Geometry: final body of the model. Coordinates: model frame, mm. Face numbers are marked on the shaded views. A direction names the side the tool comes from. Coordinates: 2 decimals unless noted, no trailing zeros. Order: outer loops, then holes, each group sorted by start corner. A loop starts at its lowest first (then second) coordinate and runs counter-clockwise, first axis right, second up. Notation, with made-up numbers: M 86.5,74 L 92.5,74 A20 ccw 92.5,98 Z; hole C 21,-1 d7. An arc over 180 degrees is marked long. Use CSV: the item, a comma, the result in double quotes. Start each with the question number.
1. First-contact query: P1, Ø17, axis at x = -33.5, y = 3, coming from the +Z side; P2, Ø6, axis at x = 8, z = 20, coming from the +Y side; P3, Ø1.5, axis at y = 3.5, z = 1.5, coming from the -X side; P4, Ø3, axis at x = 20, y = 3.05, coming from the +Z side. Flat tips, straight axial feed; report the tip coordinate or a pass-through.
2. Section query A-A on x = -20. Return the cut outline in (y, z).
3. Section query B-B on y = 7. Return the cut outline in (x, z).
4. Set-up query: the marked faces 1, 2 and 3. Return all of +Z, -Z, +X, -X, +Y, -Y with unobstructed straight access to the full face (end or side cutting, diameter ignored); none if empty.
5. Section query D-D on x = 31.5. Return the cut outline in (y, z).
6. Material intervals for line 1 (Y direction, x = 20, z = 3.5); line 2 (Y direction, x = -20, z = 3.8); line 3 (X direction, y = 20, z = 30), sorted ascending.
7. Section query C-C on z = 7.5. Return the cut outline in (x, y).
8. Pull-direction query (X, two-part tool) for the marked faces 4, 5 and 6; classes: pulls with the +X half, pulls with the -X half, needs draft (parallel to the pull), parting line crosses it, or undercut.
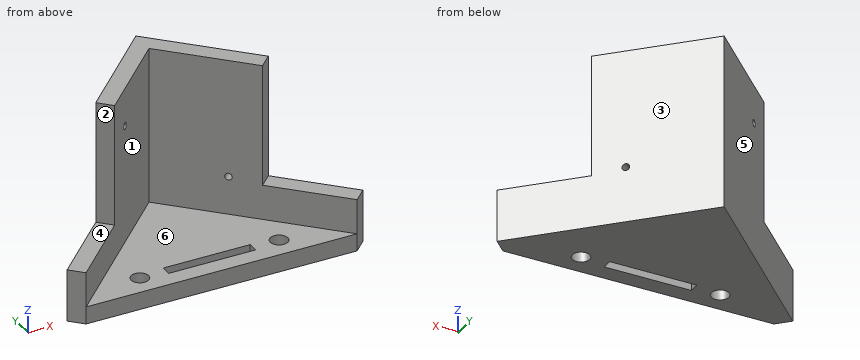
from build123d import *

# Parameters (mm, degrees)
F1_DEPTH  = 50
F3_DEPTH  = 5
F4_W      = 25
F4_H      = 3
F4_R      = 2.5
F5_DEPTH  = 25
F6_R      = 1
F8_DEPTH  = 25
F7_R      = 1
F9_DEPTH  = 25
F13_DEPTH = 35


# Not quite as in the source:
# - a feature names something its author has since deleted; it is built from what else it names


with BuildPart() as f1:
    # F0 (on Top) → F1 (new body)
    with BuildSketch(Plane.XY):
        Polygon((0, 42.4264068712), (-42.4264068712, 0), (-38.8908729653, -3.5355339059), (0, 35.3553390593), (38.8908729653, -3.5355339059), (42.4264068712, 0), align=None)
    extrude(amount=F1_DEPTH)

    # F2 (on face) → F3 (join)
    with BuildSketch(Plane(origin=(0, 0, 0), x_dir=(1, 0, 0), z_dir=(0, 0, -1))):
        Polygon((38.8908729653, 3.5355339059), (-38.8908729653, 3.5355339059), (0, -35.3553390593), align=None)
    extrude(amount=-F3_DEPTH)

    # F4 (on face) → F5 (cut)
    with BuildSketch(Plane(origin=(0, 0, 0), x_dir=(1, 0, 0), z_dir=(0, 0, -1))):
        with Locations((0, -2.9644660941)):
            Rectangle(F4_W, F4_H)
        with Locations((20, -3.0505650211)):
            Circle(F4_R)
        with Locations((-20, -2.8942257773)):
            Circle(F4_R)
    extrude(amount=-F5_DEPTH, mode=Mode.SUBTRACT)

    # F6 (on face) → F8 (cut)
    with BuildSketch(Plane(origin=(-17.6776695297, 17.6776695297, 0), x_dir=(0.7071067812, 0.7071067812, 0), z_dir=(0.7071067812, -0.7071067812, 0))):
        with Locations((4, 39)):
            Circle(F6_R)
    extrude(amount=-F8_DEPTH, mode=Mode.SUBTRACT)

    # F7 (on face) → F9 (cut)
    with BuildSketch(Plane(origin=(17.6776695297, 17.6776695297, 0), x_dir=(0.7071067812, -0.7071067812, 0), z_dir=(-0.7071067812, -0.7071067812, 0))):
        with Locations((-4, 16)):
            Circle(F7_R)
    extrude(amount=-F9_DEPTH, mode=Mode.SUBTRACT)

    # F12 (on face) → F13 (cut)
    with BuildSketch(Plane.XY.offset(50)):
        Polygon((-38.8908729653, -3.5355339059), (-21.2132034356, 14.1421356237), (-24.7487373415, 17.6776695297), (-42.4264068712, 0), align=None)
        Polygon((24.7487373415, 17.6776695297), (21.2132034356, 14.1421356237), (38.8908729653, -3.5355339059), (42.4264068712, 0), align=None)
    extrude(amount=-F13_DEPTH, mode=Mode.SUBTRACT)


solid = f1.part
Results list:
1,P1,"stops at z = 15"
1,P2,"stops at y = 37.43"
1,P3,"stops at x = -39.68"
1,P4,"passes through"
2,outline,"M -3.54,0 L 0.39,0 L 0.39,5 L -3.54,5 Z; M 5.39,0 L 22.43,0 L 22.43,50 L 15.36,50 L 15.36,5 L 5.39,5 Z"
3,outline,"M -35.43,0 L 35.43,0 L 35.43,15 L 28.36,15 L 28.36,5 L -28.36,5 L -28.36,15 L -35.43,15 Z"
4,face 1,"+Z, -Y"
4,face 2,"+Z, -X, -Y"
4,face 3,"+Z, -Z, +X, +Y"
5,outline,"M -3.54,0 L 10.93,0 L 10.93,15 L 3.86,15 L 3.86,5 L -3.54,5 Z"
6,line 1,"y = -3.54 to 0.55, 5.55 to 22.43"
6,line 2,"y = -3.54 to 0.39, 5.39 to 22.43"
6,line 3,"x = -22.43 to -15.36, 15.36 to 22.43"
7,outline,"M -42.43,0 L -38.89,-3.54 L 0,35.36 L 38.89,-3.54 L 42.43,0 L 0,42.43 Z"
8,face 4,"needs draft"
8,face 5,"pulls with the -X half"
8,face 6,"undercut"
